Part model, mm, in its own coordinate system. A direction names the side the tool comes from. Give positions to 0.01 mm unless a question says otherwise; leave off trailing zeros. Order: outer loops, then holes, each group sorted by start corner. A loop starts at its lowest first (then second) coordinate and runs counter-clockwise, first axis right, second up.
from build123d import *

# Parameters (mm, degrees)
SKETCH1_R                = 15
BOSS_EXTRUDE1_DEPTH      = 17
SKETCH2_W                = 30
SKETCH2_H                = 30
BOSS_EXTRUDE2_DEPTH      = 3
FILLET2_R                = 1
BOSS_EXTRUDE4_DEPTH      = 3
BOSS_EXTRUDE5_DEPTH      = 18
FILLET5_R                = 1
FILLET6_R                = 1
FILLET7_R                = 1
SKETCH7_R                = 14
CUT_EXTRUDE1_DEPTH       = 13
SKETCH8_R                = 1.5
CUT_EXTRUDE2_DEPTH       = 13
SKETCH9_R                = 3.5
BOSS_EXTRUDE6_DEPTH      = 1
CUT_EXTRUDE3_START       = -1
SKETCH10_R               = 1.5
CUT_EXTRUDE3_DEPTH       = 1
FILLET8_R                = 1
SKETCH13_R               = 1
CUT_EXTRUDE4_DEPTH       = 35.607752779
SKETCH14_R               = 2.5
BOSS_EXTRUDE7_DEPTH      = 30
BOSS_EXTRUDE8_DEPTH      = 16
BOSS_EXTRUDE8_DEPTH_BACK = 16
SKETCH17_R               = 4
FILLET9_R                = 2


# Some blends are built 0.0001 mm under size
with BuildPart() as part:
    # Sketch1 → Boss-Extrude1 (new body)
    with BuildSketch(Plane(origin=(0, 0, 0), x_dir=(1, 0, 0), z_dir=(0, 1, 0))):
        with Locations(Location((0, 0, 0), (0, 0, 270))):
            Circle(SKETCH1_R)
    extrude(amount=BOSS_EXTRUDE1_DEPTH)

    # Sketch2 → Boss-Extrude2 (add)
    with BuildSketch(Plane(origin=(0, 17, 0), x_dir=(1, 0, 0), z_dir=(0, 1, 0))):
        Rectangle(SKETCH2_W, SKETCH2_H)
    extrude(amount=BOSS_EXTRUDE2_DEPTH)

    # Fillet2
    fillet2_edges = [part.edges().sort_by_distance(p)[0] for p in [
        (0, 0, -15),
    ]]
    fillet(fillet2_edges, radius=FILLET2_R)

    # Sketch4 → Boss-Extrude4 (add)
    with BuildSketch(Plane(origin=(0, 20, 0), x_dir=(1, 0, 0), z_dir=(0, 1, 0))):
        Polygon((15, 15), (24.270248109, 11.25), (15, -3), align=None)
    extrude(amount=-BOSS_EXTRUDE4_DEPTH)

    # Sketch6 → Boss-Extrude5 (add)
    with BuildSketch(Plane(origin=(0, 20, 0), x_dir=(1, 0, 0), z_dir=(0, 1, 0))):
        Polygon((15, -3), (0, -3), (0, 15), (15, 15), (24.270248109, 11.25), align=None)
    extrude(amount=-BOSS_EXTRUDE5_DEPTH)

    # Fillet5
    fillet5_edges = [part.edges().sort_by_distance(p)[0] for p in [
        (15, 18.5, 3),
        (24.270248109, 11, -11.25),
        (15, 18.5, 15),
        (15, 11, -15),
        (-15, 18.5, -15),
        (-15, 18.5, 15),
    ]]
    fillet(fillet5_edges, radius=FILLET5_R)

    # Fillet6
    # the kernel refuses this fillet: 1 mm, written as the material it adds along each edge
    with BuildSketch(Plane(origin=(14.696938457, 18.556304537, 3), x_dir=(-0.2202884134263797, 0, 0.9754347824996238), z_dir=(0, -1, 0))) as fillet6_piece_1:
        with BuildLine():
            CenterArc((0.643272542, -0.99978468), FILLET6_R, 91.189014428, 44.048625674)
            Line((-0.066760947, -0.295616771), (-0.080961616, -0.281533412))
            ThreePointArc((-0.080961616, -0.281533412), (-0.052889169, -0.143402617), (-0.019508696, 0.004405768))
            Line((-0.019508696, 0.004405768), (0.000415015, 0.019995694))
            ThreePointArc((0.000415015, 0.019995694), (0.311260907, 0.016770207), (0.6221068, 0.019995694))
            Line((0.6221068, 0.019995694), (0.622521815, 0))
        make_face()
    extrude(amount=16.556304537)

    # Fillet7
    fillet7_edges = [part.edges().sort_by_distance(p)[0] for p in [
        (15, 9.5, 3),
    ]]
    fillet(fillet7_edges, radius=FILLET7_R)

    # Sketch7 → Cut-Extrude1 (cut)
    with BuildSketch(Plane(origin=(0, 20, 0), x_dir=(1, 0, 0), z_dir=(0, 1, 0))):
        with BuildLine():
            Line((14.805399496, 14), (0, 14))
            ThreePointArc((0, 14), (9.899494937, 9.899494937), (14, 0))
            ThreePointArc((14, 0), (13.900075645, -1.66969969), (13.601728992, -3.31556457))
            Line((13.601728992, -3.31556457), (22.770248109, 10.778060096))
            Line((22.770248109, 10.778060096), (14.805399496, 14))
        make_face()
        Circle(SKETCH7_R)
    extrude(amount=-CUT_EXTRUDE1_DEPTH, mode=Mode.SUBTRACT)

    # Sketch8 → Cut-Extrude2 (cut)
    with BuildSketch(Plane(origin=(7.323889561, 0, -18.105139561), x_dir=(-0.927024810886958, 0, -0.3749999999999998), z_dir=(0.3749999999999998, 0, -0.927024810886958))):
        with Locations((-12.770892539, 11)):
            Circle(SKETCH8_R)
    extrude(amount=-CUT_EXTRUDE2_DEPTH, mode=Mode.SUBTRACT)

    # Sketch9 → Boss-Extrude6 (add)
    with BuildSketch(Plane(origin=(7.323889561, 0, -18.105139561), x_dir=(-0.927024810886958, 0, -0.3749999999999998), z_dir=(0.3749999999999998, 0, -0.927024810886958))):
        with Locations((-12.770892539, 11)):
            Circle(SKETCH9_R)
    extrude(amount=BOSS_EXTRUDE6_DEPTH)

    # Sketch10 → Cut-Extrude3 (cut)
    with BuildSketch(Plane(origin=(7.323889561, 0, -18.105139561), x_dir=(0.927024810886958, 0, 0.3749999999999998), z_dir=(-0.3749999999999998, 0, 0.927024810886958)).offset(CUT_EXTRUDE3_START)):
        with Locations((12.770892539, 11)):
            Circle(SKETCH10_R)
    extrude(amount=CUT_EXTRUDE3_DEPTH, mode=Mode.SUBTRACT)

    # Fillet8
    fillet8_edges = [part.edges().sort_by_distance(p)[0] for p in [
        (22.78241064, 11, -12.93057967),
    ]]
    fillet(fillet8_edges, radius=FILLET8_R - 0.0001)  # a hair under: the kernel refuses the full size

    # Sketch13 → Cut-Extrude4 (cut, through all)
    with BuildSketch(Plane(origin=(0, 20, 0), x_dir=(1, 0, 0), z_dir=(0, 1, 0))):
        with Locations(Location((-13, 13, 0), (0, 0, 270))):
            Circle(SKETCH13_R)
        with Locations(Location((-13, -13, 0), (0, 0, 270))):
            Circle(SKETCH13_R)
        with Locations(Location((13, -13, 0), (0, 0, 270))):
            Circle(SKETCH13_R)
    extrude(amount=-CUT_EXTRUDE4_DEPTH, mode=Mode.SUBTRACT)

    # Sketch14 → Boss-Extrude7 (add)
    with BuildSketch(Plane(origin=(7.698889561, 0, -19.032164372), x_dir=(-0.927024810886958, 0, -0.3749999999999998), z_dir=(0.3749999999999998, 0, -0.927024810886958))):
        with Locations((-12.770892539, 11)):
            Circle(SKETCH14_R)
    extrude(amount=BOSS_EXTRUDE7_DEPTH)

    # Sketch17 → Boss-Extrude8 (add, two sides: drawn at the far end of the back side and taken through both)
    with BuildSketch(Plane(origin=(11.838934241, 0, 4.789084702), x_dir=(0.3749999999999998, 0, -0.927024810886958), z_dir=(0.927024810886958, 0, 0.3749999999999998)).offset(-BOSS_EXTRUDE8_DEPTH_BACK)):
        with Locations((50.530372163, 11)):
            Circle(SKETCH17_R)
    extrude(amount=BOSS_EXTRUDE8_DEPTH + BOSS_EXTRUDE8_DEPTH_BACK)

    # Fillet9
    fillet9_edges = [part.edges().sort_by_distance(p)[0] for p in [
        (14.455426828, 11, -44.345724753),
        (44.120220776, 11, -32.345724753),
    ]]
    fillet(fillet9_edges, radius=FILLET9_R)


solid = part.part
Item 1: Drill centre lines: probe 1 along Z at (x, y) = (17, 8.25); probe 2 along Y at (x, z) = (9, -2); probe 3 along Z at (x, y) = (0, 15). Where is each one in solid material? Low to high.
Item 2: Pull direction X, two halves, no side cores. Call faces 4 (the face through (-14, 19, 13)), 5 (the face through (0, 18, 15)), 6 (the face through (15.945, 11.028, -48.028)): released by +X, released by -X, zero draft, split by the parting line, or undercut.
Item 3: Band-saw the part on C-C on y = 4.5. List the corners of the cut face in (x, z), plus the area to 3 significant figures.
Item 4: Which spindle directions (+Z, -Z, +X, -X, +Y, -Y) get a long thin tool onto all of the face, cutting with end or side? Do faces 1 (the face through (15, 18, 9)), 2 (the face through (19.557, 11.021, -14.235)), 3 (the face through (-11, 17, -12)). Say none if no direction does.
Item 5: Band-saw the part on A-A on y = 15.75. List the corners of the cut face in (x, z), plus the area to 3 significant figures.
Item 6: Band-saw the part on B-B on x = -13. Give the number of separate pieces and of enclosed holes in the cut face, plus the area to 3 significant figures.
Item 7: Drop flat-ended pins along their axis: P1, Ø10, axis at y = 8, z = -14, coming from the +X side; P2, Ø3.5, axis at y = 18, z = 6.5, coming from the +X side; P3, Ø6.5, axis at x = 7, y = 13, coming from the +Z side; P4, Ø2, axis at y = 5, z = -38.5, coming from the -X side. Give the stop position or say it passes through.
Working result:
1. probe 1: z = -49.48 to -44.5, -14.19 to -13.11, -1.91 to -0.07
1. probe 2: y = 0 to 7
1. probe 3: z = -15 to -14, 14 to 15
2. face 4: undercut
2. face 5: zero draft
2. face 6: released by -X
3. outline: (0, -15) - (14.81, -15) arc R1 ccw to (15.18, -14.93) - (23.15, -11.71) arc R1 ccw to (23.61, -10.23) - (15.1, 2.85) arc R1 ccw to (14.9, 3.08) arc R1 cw to (14.56, 3.61) arc R15 ccw (long way) to start
3. area: 839 mm2
4. face 1: +Z, +X, +Y, -Y
4. face 2: none
4. face 3: -Z, -X, -Y
5. outline: (0, -15) - (14.81, -15) arc R1 ccw to (15.18, -14.93) - (23.15, -11.71) arc R1 ccw to (23.61, -10.23) - (15.1, 2.85) arc R1 ccw to (14.9, 3.08) arc R1 cw to (14.56, 3.61) arc R15 ccw (long way) to start; hole (0, -14) - (14.81, -14) - (22.77, -10.78) - (13.6, 3.32) arc R14 ccw (long way) to start
5. area: 106 mm2
6. separate pieces: 3
6. enclosed holes: 0
6. area: 196 mm2
7. P1: stops at x = 23.83
7. P2: stops at x = 15
7. P3: stops at z = 14.52
7. P4: passes through
